from build123d import *

# Parameters (mm, degrees)
SKETCH1_W           = 107
SKETCH1_H           = 86
BOSS_EXTRUDE1_DEPTH = 2
FILLET1_R           = 10
SKETCH5_R           = 7.5
CUT_EXTRUDE1_DEPTH  = 2


# Read off the part's stored shape, not the designer's step: Shell2
with BuildPart() as part:
    # Sketch1 → Boss-Extrude1 (new body)
    with BuildSketch(Plane.XY):
        Rectangle(SKETCH1_W, SKETCH1_H)
        with BuildLine():
            Line((-43, 34), (-40, 34))
            ThreePointArc((-40, 34), (-36, 30), (-40, 26))
            Line((-40, 26), (-43, 26))
            ThreePointArc((-43, 26), (-47, 30), (-43, 34))
        make_face(mode=Mode.SUBTRACT)
        with BuildLine():
            Line((43, 34), (40, 34))
            ThreePointArc((40, 34), (36, 30), (40, 26))
            Line((40, 26), (43, 26))
            ThreePointArc((43, 26), (47, 30), (43, 34))
        make_face(mode=Mode.SUBTRACT)
        with BuildLine():
            Line((43, -34), (40, -34))
            ThreePointArc((40, -34), (36, -30), (40, -26))
            Line((40, -26), (43, -26))
            ThreePointArc((43, -26), (47, -30), (43, -34))
        make_face(mode=Mode.SUBTRACT)
        with BuildLine():
            Line((-43, -34), (-40, -34))
            ThreePointArc((-40, -34), (-36, -30), (-40, -26))
            Line((-40, -26), (-43, -26))
            ThreePointArc((-43, -26), (-47, -30), (-43, -34))
        make_face(mode=Mode.SUBTRACT)
    extrude(amount=BOSS_EXTRUDE1_DEPTH)

    # Fillet1
    fillet1_edges = [part.edges().sort_by_distance(p)[0] for p in [
        (-53.5, 43, 1),
        (53.5, 43, 1),
        (53.5, -43, 1),
        (-53.5, -43, 1),
    ]]
    fillet(fillet1_edges, radius=FILLET1_R)

    # Sketch3 → Revolve1 (revolve)
    with BuildSketch(Plane(origin=(0, 0, 0), x_dir=(1, 0, 0), z_dir=(0, 1, 0)), mode=Mode.PRIVATE) as revolve1_sk:
        Polygon((37.75, -2), (34.294777143, -5), (20.75, -5), (14.991295238, -10), (0, -10), (0, -2), align=None)
    revolve(revolve1_sk.sketch.rotate(Axis((0, 0, 0), (0, 0, 1)), 180), axis=Axis((0, 0, 0), (0, 0, 1)))

    # Shell2 outline → Shell2 (revolve, cut)
    with BuildSketch(Plane.XZ):
        Polygon((37, 0), (37, 0.002520926), (33.547680597, 3), (20.002903454, 3), (14.244198692, 8), (0, 8), (0, 0), align=None)
    revolve(axis=Axis((0, 0, 0), (0, 0, 1)), mode=Mode.SUBTRACT)

    # Sketch5 → Cut-Extrude1 (cut)
    with BuildSketch(Plane.XY.offset(10)):
        Circle(SKETCH5_R)
    extrude(amount=-CUT_EXTRUDE1_DEPTH, mode=Mode.SUBTRACT)


solid = part.part
Verification items for the finished model (mm, model axes). A direction names the side the tool comes from. Give positions to 0.01 mm unless a question says otherwise; leave off trailing zeros. Write each loop counter-clockwise with the first axis right and the second up, starting at its lowest first coordinate (ties: lowest second). Pieces come first, ordered by that corner, then holes. Notation, with made-up numbers: M 67,55 L 117,55 A25 cw 117,83 Z; hole C 31,-37 d1. An arc over 180 degrees is marked long. Use CSV: the item, a comma, the result in double quotes.
1) Go/stop test with flat-tipped pins: pin 1 Ø3 at (y, z) = (-12.5, 8) entering from -X (3 decimals); pin 2 Ø6 at (x, y) = (-31, 8.5) entering from +Z; pin 3 Ø20 at (x, y) = (-12.5, -8) entering from -Z. Record where each tip stops, or that it passes through.
Final values:
pin 1,"x = -14.665"
pin 2,"z = 5"
pin 3,"z = 3"
2) Access from +Z, -Z, +X, -X, +Y, -Y to the whole of each face (thin tool, end or side, straight path). Record for faces 5 (the face through (-36, 30, 1)), 6 (the face through (-50.65, -39.99, 1.01)).
Final values:
face 5,"+Z, -Z"
face 6,"+Z, -Z, -X, -Y"
3) Cross-section at B-B (z = 6.75). Enter the section's corners in (x, y).
Final values:
outline,"C 0,0 d37.47; hole C 0,0 d31.37"
4) Cross-section at C-C (y = -30). State how many separate pieces and enclosed holes the cut face has, plus the area to 3 significant figures.
Final values:
separate pieces,"3"
enclosed holes,"0"
area,"178 mm²"
5) Release check for a two-part mould opening along X. For faces 1 (the face through (-15, 15, 5)), 2 (the face through (-50.65, 39.99, 1.01)), 3 (the face through (6, -6, 8)), 4 (the face through (-7.493, 0.33, 9.014)) record: released by +X, released by -X, zero draft, split by the parting line, or undercut.
Final values:
face 1,"zero draft"
face 2,"released by -X"
face 3,"undercut"
face 4,"undercut"
6) Material ranges on line 1 along Z through (x, y) = (16, -37.5); line 2 along Y through (x, z) = (-5.5, 4); line 3 along Y through (x, z) = (0, 9.55), recorded low to high.
Final values:
line 1,"0 to 2"
line 2,"-35.02 to -18.03, 18.03 to 35.02"
line 3,"-15.51 to -7.5, 7.5 to 15.51"
